Here's the drawing with two shaded views (mm, measured from the low corner). I have some questions. A direction names the side the tool comes from. Round coordinates to 2 decimals unless told otherwise and drop trailing zeros. Write each loop counter-clockwise with the first axis right and the second up, starting at its lowest first coordinate (ties: lowest second). Pieces come first, ordered by that corner, then holes. Notation, with made-up numbers: M 3.25,17 L 13.25,17 A17 cw 13.25,44 Z; hole C 62.25,-21 d3. An arc over 180 degrees is marked long. Answer as a JSON object with one key per item and string values. Group by question number.
1) Please list where these lines run through material, in increasing order: L1, parallel to X at y = 6.25, z = 4.55; L2, parallel to Z at x = 30, y = 7. Write a range as [from, to].
2) I'm going to push flat-ended pins straight in: pin 1 Ø2.5 at (y, z) = (3.5, 2.5) entering from -X; pin 2 Ø1 at (x, y) = (38, 3) entering from +Z. Where does each tip first touch, or does it pass through?
3) Suppose I cut it at A-A, the plane z = 2.6. Write out the boundary of the cut face in (x, y), and give its area (3 significant figures).
4) On a 3-axis mill with a long thin cutter (end or side, diameter ignored), from which of +Z, -Z, +X, -X, +Y, -Y can I reach the whole of each face in a straight line? I mean the marked faces 3 and 4. Say none if no direction works.
5) Suppose I cut it at B-B, the plane y = 5.25. Write out the boundary of the cut face in (x, z).
6) Suppose I cut it at C-C, the plane x = 25.5. Write out the boundary of the cut face in (y, z), and give its area (3 significant figures).
7) If we mould it in two halves opening along X, with no side actions, what happens to the marked faces 1 and 2? For each: +X half, -X half, draft (parallel to the pull), parting line (faces both ways), or undercut.
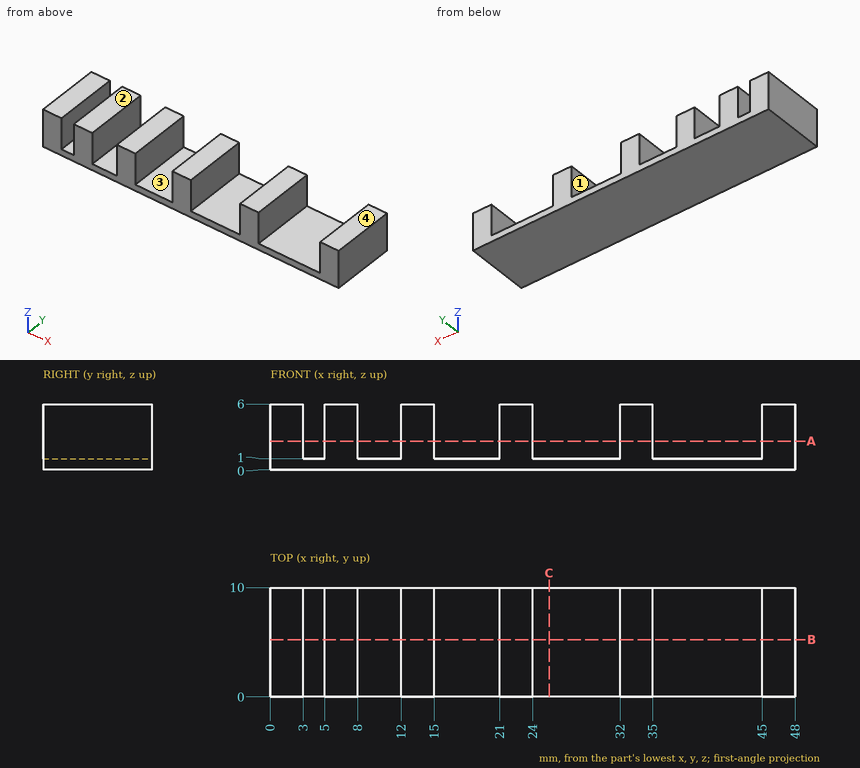
Results:
{
 "1": {"L1": "[0, 3], [5, 8], [12, 15], [21, 24], [32, 35], [45, 48]", "L2": "[0, 1]"},
 "2": {"pin 1": "x = 0", "pin 2": "z = 1"},
 "3": {"outline": "M 0,0 L 3,0 L 3,10 L 0,10 Z; M 5,0 L 8,0 L 8,10 L 5,10 Z; M 12,0 L 15,0 L 15,10 L 12,10 Z; M 21,0 L 24,0 L 24,10 L 21,10 Z; M 32,0 L 35,0 L 35,10 L 32,10 Z; M 45,0 L 48,0 L 48,10 L 45,10 Z", "area": "180 mm^2"},
 "4": {"face 3": "+Z, +Y, -Y", "face 4": "+Z, +X, -X, +Y, -Y"},
 "5": {"outline": "M 0,0 L 48,0 L 48,6 L 45,6 L 45,1 L 35,1 L 35,6 L 32,6 L 32,1 L 24,1 L 24,6 L 21,6 L 21,1 L 15,1 L 15,6 L 12,6 L 12,1 L 8,1 L 8,6 L 5,6 L 5,1 L 3,1 L 3,6 L 0,6 Z"},
 "6": {"outline": "M 0,0 L 10,0 L 10,1 L 0,1 Z", "area": "10.0 mm^2"},
 "7": {"face 1": "undercut", "face 2": "draft"}
}
